Autodesk Inventor part; units mm, degrees
ref_plane "工作平面1" through (10, 18, 0) normal (-0.3716, -0.6565, -0.6565) x (0.8703, 0, -0.4926)
ref_plane "YZ Plane" through (0, 0, 0) normal (1, 0, 0) x (0, 1, 0)
ref_plane "XZ Plane" through (0, 0, 0) normal (0, 1, 0) x (-1, 0, 0)
sketch "草圖1" plane through (0, 0, 0) normal (0, 1, 0) x (-1, 0, 0)
  line L0 (0, 0) -> (-63, 0)
  line L1 (-63, 0) -> (-63, -40)
  line L2 (-63, -40) -> (0, -40)
  line L3 (0, -40) -> (0, 0)
  dimension "d0" = 63
  dimension "d1" = 40
extrude "擠出1" add sketch "草圖1" along normal mid plane 36
sketch "草圖2" plane through (0, 18, 0) normal (0, 1, 0) x (1, 0, 0)
  line L0 (0, 0) -> (63, 0)
  line L1 (10, 0) -> (63, 10)
  line L2 (63, 0) -> (63, 40)
  dimension "d4" = 10
  dimension "d5" = 30
extrude "擠出2" cut sketch "草圖2" against normal blind 40
sketch "草圖3" plane through (63, -18, -40) normal (1, 0, 0) x (0, 0, -1)
  line L0 (-30, 16) -> (-10, 36)
  line L1 (0, 36) -> (-40, 36)
  line L2 (-30, 36) -> (-30, 0)
  point P0 (-40, 18)
  dimension "d8" = 20
  dimension "d9" = 20
ref_plane "工作平面1" through (10, 18, 0) normal (-0.3716, -0.6565, -0.6565) x (0.8703, 0, -0.4926)
sketch "草圖4" plane through (10, 18, 0) normal (-0.3716, -0.6565, -0.6565) x (0.8703, 0, -0.4926)
  line L0 (-15.1543, -12.3218) -> (93.717, -12.3218)
  line L1 (93.717, -12.3218) -> (93.717, 28.8166)
  line L2 (93.717, 28.8166) -> (-15.1543, 28.8166)
  line L3 (-15.1543, 28.8166) -> (-15.1543, -12.3218)
  point P0 (-8.7026, 10.3445)
extrude "擠出3" cut sketch "草圖4" against normal blind 40
mirror "鏡射1" about plane through (0, 0, 0) normal (0, 1, 0) of "擠出3"
properties part number "14"
CAD build for the part. Positions are in the model's coordinates, mm. Give positions to 0.01 mm unless a question says otherwise; leave off trailing zeros. Loops run counter-clockwise (first coordinate to the right, second up) from the corner with the lowest first, then second, coordinate; pieces in that order, holes last. Notation, with made-up numbers: M 78.25,-21 L 126.25,-21 A17 ccw 126.25,9 Z; hole C -36,51.5 d8. An arc over 180 degrees is marked long. One line per question, with ' | ' between items. Start each with the question number.
1. Saw through at A-A on y = 11.5. Give the cut face in (x, z).
2. Probe L1, parallel to Z at x = 43.5, y = 3; L2, parallel to X at y = 15.5, z = -7.5; L3, parallel to X at y = -15, z = -21. List the from-to ranges inside material, lowest first. Write a range as from..to.
3. Saw through at B-B on x = 23. Give the cut face in (y, z), plus the area to 3 significant figures.
Result sheet:
1) outline: M 0,-40 L 63,-40 L 63,-23.5 L 27.22,-3.25 L 10,0 L 0,0 Z
2) L1: z = -40..-6.32 | L2: x = 0..27.66 | L3: x = 0..52.4
3) outline: M -18,-40 L 18,-40 L 18,-7.36 L 13.09,-2.45 L -13.09,-2.45 L -18,-7.36 Z | area: 1,330 mm^2
